The model under review builds one solid part; all positions refer to its coordinate system, in mm. A direction names the side the tool comes from. Give positions to 0.01 mm unless a question says otherwise; leave off trailing zeros. Order: outer loops, then holes, each group sorted by start corner. A loop starts at its lowest first (then second) coordinate and runs counter-clockwise, first axis right, second up.
```python
from build123d import *

# Parameters (mm, degrees)
ESQUISSE2_R             = 2.5
ESQUISSE2_R_2           = 1.5
ENL_V_MAT_EXTRU_1_DEPTH = 10


with BuildPart() as part:
    # Esquisse1 → Révolution1 (revolve)
    with BuildSketch(Plane.XY):
        Polygon((0, 0), (0, 11), (0.5, 11), (1, 10), (3, 10), (3.5, 11), (4, 11), (4, 0), align=None)
    revolve(axis=Axis((4, 0, 0), (-1, 0, 0)))

    # Esquisse2 → Enlèv. mat.-Extru.1 (cut)
    with BuildSketch(Plane(origin=(4, 0, 0), x_dir=(0, 0, -1), z_dir=(1, 0, 0))):
        with Locations(Location((0, 0, 0), (0, 0, 90))):
            Circle(ESQUISSE2_R)
        with Locations(Location((0, 7, 0), (0, 0, 90))):
            Circle(ESQUISSE2_R_2)
        with Locations(Location((0, -7, 0), (0, 0, 90))):
            Circle(ESQUISSE2_R_2)
    extrude(amount=-ENL_V_MAT_EXTRU_1_DEPTH, mode=Mode.SUBTRACT)


solid = part.part
```
Item 1: Take a section at B-B (y = 0). Give the boundary of the cut face in (x, z).
Values found:
outline: (0, -11) - (0.5, -11) - (1, -10) - (3, -10) - (3.5, -11) - (4, -11) - (4, -2.5) - (0, -2.5) - close; (0, 2.5) - (4, 2.5) - (4, 11) - (3.5, 11) - (3, 10) - (1, 10) - (0.5, 11) - (0, 11) - close
Item 2: Draft analysis for pull direction Z (two halves, no side actions). For faces 1 (the cylindrical face through (2.03, 5.5, 0.07)), 2 (the cylindrical face through (3.75, -2.38, 10.74)), 3 (the flat face through (4, 0, -3)), state which applies: released by +Z, released by -Z, zero draft, split by the parting line, or undercut.
Values found:
face 1: undercut
face 2: split by the parting line
face 3: zero draft
Item 3: Take a section at A-A (z = 0). Give the boundary of the cut face in (x, y), and give its area (3 significant figures).
Values found:
outline: (0, -11) - (0.5, -11) - (1, -10) - (3, -10) - (3.5, -11) - (4, -11) - (4, -8.5) - (0, -8.5) - close; (0, -5.5) - (4, -5.5) - (4, -2.5) - (0, -2.5) - close; (0, 2.5) - (4, 2.5) - (4, 5.5) - (0, 5.5) - close; (0, 8.5) - (4, 8.5) - (4, 11) - (3.5, 11) - (3, 10) - (1, 10) - (0.5, 11) - (0, 11) - close
area: 39.0 mm2
Item 4: Take a section at C-C (x = 1.3). Give the boundary of the cut face in (y, z), and give its area (3 significant figures).
Values found:
outline: circle Ø20 at (0, 0); hole circle Ø3 at (-7, 0); hole circle Ø5 at (0, 0); hole circle Ø3 at (7, 0)
area: 280 mm2
Item 5: For line 1 (Z direction, x = 1.3, y = 0); line 2 (Z direction, x = 0.7, y = 0.5); line 3 (X direction, y = 3, z = 9.75), list the stretches that pass through material, from the lowest coordinate up.
Values found:
line 1: z = -10 to -2.5, 2.5 to 10
line 2: z = -10.59 to -2.45, 2.45 to 10.59
line 3: x = 0 to 0.9, 3.1 to 4
Item 6: Clearance check with a flat-ended pin moving along its axis: pin 1 Ø2 at (x, z) = (3, 4) entering from +Y. State where the tip first meets the part, or that it passes through.
Values found:
pin 1: stops at y = 10.54
Item 7: For faces 4 (the cylindrical face through (0.25, -2.38, 10.74)), 5 (the cylindrical face through (2.01, -2.17, 9.76)), list the 3-axis set-ups (+Z, -Z, +X, -X, +Y, -Y) from which the entire face can be reached by the end or side of a thin tool; tool diameter is ignored.
Values found:
face 4: +X, -X
face 5: none
